from build123d import *

# Parameters (mm, degrees)
SKETCH3_R           = 195
SKETCH3_R_2         = 150
BOSS_EXTRUDE3_START = -45
SKETCH8_W           = 500
SKETCH8_H           = 500
SKETCH8_R           = 195
BOSS_EXTRUDE3_DEPTH = 45
FILLET3_R           = 10
SKETCH9_W           = 500
SKETCH9_H           = 500
SKETCH9_R           = 195
BOSS_EXTRUDE4_DEPTH = 45
FILLET4_R           = 10
CUT_EXTRUDE2_REACH  = 818.211
SKETCH10_R          = 32.5
CIRPATTERN2_COUNT   = 4
CUT_EXTRUDE3_REACH  = 968.282
SKETCH11_R          = 32.5
CIRPATTERN3_COUNT   = 4


with BuildPart() as part:
    # Sweep-Thin4: sweep along a path in Sketch2
    with BuildLine(Plane.XY) as sweep_thin4_path:
        Line((0, 0), (-160, 0))
        ThreePointArc((-160, 0), (-336.776695297, 73.223304703), (-410, 250))
        Line((-410, 250), (-410, 410))
    # Sketch3 → Sweep-Thin4 (sweep)
    with BuildSketch(Plane(origin=(0, 0, 0), x_dir=(0, 0, -1), z_dir=(1, 0, 0))):
        Circle(SKETCH3_R)
        Circle(SKETCH3_R_2, mode=Mode.SUBTRACT)
    sweep(path=sweep_thin4_path.line)

    # Sketch8 → Boss-Extrude3 (add)
    with BuildSketch(Plane(origin=(0, 0, 0), x_dir=(0, 0, -1), z_dir=(1, 0, 0)).offset(BOSS_EXTRUDE3_START)):
        Rectangle(SKETCH8_W, SKETCH8_H)
        with Locations(Location((0, 0, 0), (0, 0, 270))):
            Circle(SKETCH8_R, mode=Mode.SUBTRACT)
    extrude(amount=BOSS_EXTRUDE3_DEPTH)

    # Fillet3
    fillet3_edges = [part.edges().sort_by_distance(p)[0] for p in [
        (-22.5, 250, -250),
        (-22.5, -250, -250),
        (-22.5, -250, 250),
        (-22.5, 250, 250),
    ]]
    fillet(fillet3_edges, radius=FILLET3_R)

    # Sketch9 → Boss-Extrude4 (add)
    with BuildSketch(Plane(origin=(0, 410, 0), x_dir=(1, 0, 0), z_dir=(0, 1, 0))):
        with Locations((-410, 0)):
            Rectangle(SKETCH9_W, SKETCH9_H)
        with Locations(Location((-410, 0, 0), (0, 0, 270))):
            Circle(SKETCH9_R, mode=Mode.SUBTRACT)
    extrude(amount=-BOSS_EXTRUDE4_DEPTH)

    # Fillet4
    fillet4_edges = [part.edges().sort_by_distance(p)[0] for p in [
        (-660, 387.5, -250),
        (-160, 387.5, -250),
        (-160, 387.5, 250),
        (-660, 387.5, 250),
    ]]
    fillet(fillet4_edges, radius=FILLET4_R)

    # Sketch10 → Cut-Extrude2 (cut, up to next)
    with BuildSketch(Plane(origin=(0, 0, 0), x_dir=(0, 0, -1), z_dir=(1, 0, 0)), mode=Mode.PRIVATE) as cut_extrude2_sk1:
        with Locations((-200, 200)):
            Circle(SKETCH10_R)
    cut_extrude2_tool1 = extrude(cut_extrude2_sk1.sketch, amount=-CUT_EXTRUDE2_REACH, mode=Mode.PRIVATE) & part.part
    cut_extrude2 = cut_extrude2_tool1.solids().sort_by_distance((0, 200, 200))[0]
    add(cut_extrude2, mode=Mode.SUBTRACT)

    # CirPattern2: Cut-Extrude2 ×4 about axis
    cirpattern2_axis = Axis((0, 0, 0), (1, 0, 0))
    for i in range(1, CIRPATTERN2_COUNT):
        add(cut_extrude2.rotate(cirpattern2_axis, i * 360 / CIRPATTERN2_COUNT), mode=Mode.SUBTRACT)

    # Sketch11 → Cut-Extrude3 (cut, up to next)
    with BuildSketch(Plane(origin=(0, 410, 0), x_dir=(1, 0, 0), z_dir=(0, 1, 0)), mode=Mode.PRIVATE) as cut_extrude3_sk1:
        with Locations(Location((-610, 200, 0), (0, 0, 270))):
            Circle(SKETCH11_R)
    cut_extrude3_tool1 = extrude(cut_extrude3_sk1.sketch, amount=-CUT_EXTRUDE3_REACH, mode=Mode.PRIVATE) & part.part
    cut_extrude3 = cut_extrude3_tool1.solids().sort_by_distance((-610, 410, -200))[0]
    add(cut_extrude3, mode=Mode.SUBTRACT)

    # CirPattern3: Cut-Extrude3 ×4 about axis
    cirpattern3_axis = Axis((-410, 0, 0), (0, 1, 0))
    for i in range(1, CIRPATTERN3_COUNT):
        add(cut_extrude3.rotate(cirpattern3_axis, i * 360 / CIRPATTERN3_COUNT), mode=Mode.SUBTRACT)


solid = part.part
Can you work these out from the model? Positions are in its coordinate system, mm. A direction names the side the tool comes from. Coordinates: 2 decimals unless noted, no trailing zeros. Loops run counter-clockwise (first coordinate to the right, second up) from the corner with the lowest first, then second, coordinate; pieces in that order, holes last. Notation, with made-up numbers: (-18.75, 81.25) - (21.25, 81.25) arc R29 ccw to (21.25, 109.25) - close; hole circle Ø11 at (16.25, 29). An arc over 180 degrees is marked (long way). Answer as a JSON object with one key per item and string values. Group by question number.
Item 1: If we mould it in two halves opening along Y, with no side actions, what happens to faces 1 (the face through (-525, 410, -115)), 2 (the face through (-23, -3, -250)), 3 (the face through (-22.18, -185, 171.17))? For each: released by +Y, released by -Y, zero draft, split by the parting line, or undercut.
Item 2: On a 3-axis mill with a long thin cutter (end or side, diameter ignored), from which of +Z, -Z, +X, -X, +Y, -Y can I reach the whole of each face in a straight line? I mean faces 4 (the face through (-22.18, 169.98, -187.55)), 5 (the face through (-45, 170, 115)), 6 (the face through (-23, 250, 3)). Say none if no direction works.
Item 3: If we section it at C-C (y = 184.5): State how many separate pieces and enclosed holes the cut face has, plus the area to 3 significant figures.
Item 4: If I drill on L1, parallel to Y at x = -18.5, z = -200; L2, parallel to X at y = 399, z = 200, over which ranges is the centre line in solid material (lowest first)? Write a range as from..to.
Item 5: For pin 1 (1.5 mm diameter, centred on x = -114.5, z = 36.5, fed in from +Y); pin 2 (3 mm diameter, centred on x = -427, y = 129, fed in from -Z); pin 3 (6 mm diameter, centred on x = -387.5, y = 7.5, fed in from +Z); pin 4 (5 mm diameter, centred on y = 114.5, z = -164.5, fed in from +X), each with a flat end and sliding along its axis, tell me the tip position at first contact or that it passes through.
Item 6: If we section it at D-D (z = 70): List the corners of the cut face in (x, y) for me (1 decimal).
Item 7: If we section it at A-A (z = 0): List the corners of the cut face in (x, y) for me, plus the area to 3 significant figures.
Item 8: If we section it at B-B (y = 326): List the corners of the cut face in (x, z) for me, plus the area to 3 significant figures.
Returned:
{
 "1": {"face 1": "released by +Y", "face 2": "zero draft", "face 3": "undercut"},
 "2": {"face 4": "+X", "face 5": "none", "face 6": "+Z, -Z, +X, +Y"},
 "3": {"separate pieces": "3", "enclosed holes": "1", "area": "88,900 mm²"},
 "4": {"L1": "y = -250..-232.5, -167.5..167.5, 232.5..250", "L2": "x = -660..-642.5, -577.5..-242.5, -177.5..-160"},
 "5": {"pin 1": "stops at y = 191.69", "pin 2": "stops at z = -190.5", "pin 3": "stops at z = 178.05", "pin 4": "stops at x = 0"},
 "6": {"outline": "(-660, 365) - (-592, 365) - (-592, 250) arc R432 ccw to (-160, -182) - (-45, -182) - (-45, -250) - (0, -250) - (0, -132.7) - (-160, -132.7) arc R382.7 cw to (-542.7, 250) - (-542.7, 410) - (-660, 410) - close; (-277.3, 250) arc R117.3 ccw to (-160, 132.7) - (0, 132.7) - (0, 250) - (-45, 250) - (-45, 182) - (-160, 182) arc R68 cw to (-228, 250) - (-228, 365) - (-160, 365) - (-160, 410) - (-277.3, 410) - close"},
 "7": {"outline": "(-660, 365) - (-605, 365) - (-605, 250) arc R445 ccw to (-160, -195) - (-45, -195) - (-45, -250) - (0, -250) - (0, -150) - (-160, -150) arc R400 cw to (-560, 250) - (-560, 410) - (-660, 410) - close; (-260, 250) arc R100 ccw to (-160, 150) - (0, 150) - (0, 250) - (-45, 250) - (-45, 195) - (-160, 195) arc R55 cw to (-215, 250) - (-215, 365) - (-160, 365) - (-160, 410) - (-260, 410) - close", "area": "74,000 mm²"},
 "8": {"outline": "circle Ø390 at (-410, 0); hole circle Ø300 at (-410, 0)", "area": "48,800 mm²"}
}
